Geometry check sheet. Reference: the model listing, model coordinates, mm. A direction names the side the tool comes from. Give positions to 0.01 mm unless a question says otherwise; leave off trailing zeros. Write each loop counter-clockwise with the first axis right and the second up, starting at its lowest first coordinate (ties: lowest second). Pieces come first, ordered by that corner, then holes. Notation, with made-up numbers: (16.5, -20) - (24.5, -20) arc R20 cw to (24.5, 15) - close; hole circle Ø10 at (89, 64). An arc over 180 degrees is marked (long way). One line per question, with ' | ' between items. Start each with the question number.
Q1. Release check for a two-part mould opening along Z. For faces 1 (the face through (-2.96, -2.46, -5.22)), 2 (the face through (2.685, -8.112, -0.596)), 3 (the face through (-3, 0, 0)) record: +Z half, -Z half, draft (parallel to the pull), parting line (faces both ways), or undercut.
Q2. Set-up check for faces 4 (the face through (3.042, -2.465, -5.172)), 5 (the face through (-5, -5, 2)): record each of +Z, -Z, +X, -X, +Y, -Y from which the full face is reachable in a straight line by a thin tool's end or side.
Q3. Gauge pin test, flat ends, axial feed: P1, Ø2, axis at x = 0.5, y = -3, coming from the +Z side; P2, Ø5, axis at y = -7.5, z = -5, coming from the +X side; P3, Ø5, axis at x = -3, y = -11.5, coming from the -Z side. Record the tip position at first contact, or that the pin passes through.
Q4. Thickness scan on L1, parallel to X at y = -4.5, z = 0; L2, parallel to X at y = -7.5, z = 0; L3, parallel to Z at x = -1.75, y = -6.75. Record the ranges inside material, lowest first. Write a range as [from, to].
Q5. Section check A-A on z = -5.5. Record the boundary of the cut face in (x, y), and give its area (3 significant figures).
```python
from build123d import *

# Parameters (mm, degrees)
RESSALTO_EXTRUS_O1_DEPTH = 5
ESBO_O2_R                = 4
RESSALTO_EXTRUS_O2_DEPTH = 11
ESBO_O3_R                = 2.75
CORTE_EXTRUS_O1_DEPTH    = 22


with BuildPart() as part:
    # Esboço1 → Ressalto-extrusão1 (new body)
    with BuildSketch(Plane(origin=(0, 0, 0), x_dir=(1, 0, 0), z_dir=(0, 1, 0))):
        Polygon((0, -6.92820323), (6, -3.464101615), (6, 3.464101615), (0, 6.92820323), (-6, 3.464101615), (-6, -3.464101615), align=None)
    extrude(amount=-RESSALTO_EXTRUS_O1_DEPTH)


with BuildPart() as body_2:
    # Esboço2 → Ressalto-extrusão2 (new body)
    with BuildSketch(Plane.XZ.offset(5)):
        with Locations(Location((0, 0, 0), (0, 0, 270))):
            Circle(ESBO_O2_R)
    extrude(amount=RESSALTO_EXTRUS_O2_DEPTH)


with BuildPart() as corte_extrus_o1_tool:
    # Esboço3 → Corte-extrusão1 (new body)
    with BuildSketch(Plane.XZ.offset(16)):
        with Locations(Location((0, 0, 0), (0, 0, 90))):
            Circle(ESBO_O3_R)
    extrude(amount=-CORTE_EXTRUS_O1_DEPTH)


with BuildPart() as part_1:
    add(part.part)

    # Corte-extrusão1: cut by corte_extrus_o1_tool
    add(corte_extrus_o1_tool.part, mode=Mode.SUBTRACT)



with BuildPart() as body_2_1:
    add(body_2.part)

    # Corte-extrusão1: cut by corte_extrus_o1_tool
    add(corte_extrus_o1_tool.part, mode=Mode.SUBTRACT)


with BuildPart() as part_2:
    add(part_1.part)

    add(body_2_1.part)  # Varredura1 merges body 2
    # Varredura1: sweep along a curve in space
    with BuildLine() as varredura1_path:
        ThreePointArc((0, -16, -4), (2.828427125, -16, -2.828427125), (4, -16, 0))
        ThreePointArc((4, -16, 0), (2.828427125, -16, 2.828427125), (0, -16, 4))
        ThreePointArc((0, -16, 4), (-2.828427125, -16, 2.828427125), (-4, -16, 0))
        ThreePointArc((-4, -16, 0), (-2.828427125, -16, -2.828427125), (0, -16, -4))
    # 3DSketch3 → Varredura1 (sweep)
    with BuildSketch(Plane(origin=(3.994740422, -5, -0.205058439), x_dir=(0.00013207405092369588, -0.999996124817467, 0.0027808104024168727), z_dir=(0, 0.0027808104266704827, 0.9999961335392108))):
        Polygon((0, 0), (0.000151027, 1.14349999), (11.000042627, 0), align=None)
    sweep(path=varredura1_path.line)


solid = part_2.part
```
Working result:
1) face 1: -Z half | face 2: undercut | face 3: draft
2) face 4: -Z, +X, +Y, -Y | face 5: -Y
3) P1: stops at z = 6.93 | P2: stops at x = 4.22 | P3: stops at z = -4.52
4) L1: x = [-6, -2.75], [2.75, 6] | L2: x = [-4.88, -2.75], [2.75, 4.88] | L3: z = [-4.64, -2.12], [2.12, 4.64]
5) outline: (-2.47, -5) - (2.47, -5) - (2.47, 0) - (-2.47, 0) - close | area: 24.7 mm2
